```python
from build123d import *

# Parameters (mm, degrees)
F0_W     = 89.995448
F0_H     = 99.06
F1_DEPTH = 38.1
F2_W     = 75.08048
F2_H     = 20.982087
F2_H_2   = 20.982086
F3_DEPTH = 38.1
F4_R     = 5.08
F5_W     = 59.154313
F5_H     = 38.1
F6_DEPTH = 10.16
F7_R     = 5.08
F8_W     = 63.199052
F8_H     = 38.1
F9_DEPTH = 7.62
F10_R    = 5.08


with BuildPart() as f1:
    # F0 (on Top) → F1 (new body)
    with BuildSketch(Plane.XY):
        with Locations((-3.918344, -0.650048)):
            Rectangle(F0_W, F0_H)
    extrude(amount=F1_DEPTH)

    # F2 (on face) → F3 (cut)
    with BuildSketch(Plane.XY.offset(38.1)):
        with Locations((-4.297534, 23.257251)):
            Rectangle(F2_W, F2_H)
        with Locations((-4.297534, -1.516776)):
            Rectangle(F2_W, F2_H_2)
        with Locations((-4.297534, -25.785215)):
            Rectangle(F2_W, F2_H)
    extrude(amount=-F3_DEPTH, mode=Mode.SUBTRACT)

    # F4
    f4_edges = [f1.edges().sort_by_distance(p)[0] for p in [
        (33.242706, 33.748295, 19.05),
        (33.242706, 8.974267, 19.05),
        (33.242706, -15.294172, 19.05),
        (-41.837774, 33.748295, 19.05),
        (-41.837774, 8.974267, 19.05),
        (-41.837774, -15.294172, 19.05),
        (-41.837774, -36.276259, 19.05),
        (-41.837774, -12.007819, 19.05),
        (-41.837774, 12.766208, 19.05),
        (33.242706, -36.276259, 19.05),
        (33.242706, -12.007819, 19.05),
        (33.242706, 12.766208, 19.05),
    ]]
    fillet(f4_edges, radius=F4_R)

    # F5 (on face) → F6 (cut)
    with BuildSketch(Plane(origin=(0, 48.879952, 0), x_dir=(-1, 0, 0), z_dir=(0, 1, 0))):
        with Locations((3.412747, 19.05)):
            Rectangle(F5_W, F5_H)
    extrude(amount=-F6_DEPTH, mode=Mode.SUBTRACT)

    # F7
    f7_edges = [f1.edges().sort_by_distance(p)[0] for p in [
        (-32.989904, 38.719952, 19.05),
        (26.164409, 38.719952, 19.05),
    ]]
    fillet(f7_edges, radius=F7_R)

    # F8 (on face) → F9 (cut)
    with BuildSketch(Plane.XZ.offset(50.180048)):
        with Locations((-2.907156, 19.05)):
            Rectangle(F8_W, F8_H)
    extrude(amount=-F9_DEPTH, mode=Mode.SUBTRACT)

    # F10
    f10_edges = [f1.edges().sort_by_distance(p)[0] for p in [
        (28.69237, -42.560048, 19.05),
        (-34.506682, -42.560048, 19.05),
    ]]
    fillet(f10_edges, radius=F10_R)


solid = f1.part
```
Source: CAD feature listing. Evaluate the final solid. Frame: model axes, mm. A direction names the side the tool comes from. Round coordinates to 2 decimals unless told otherwise and drop trailing zeros. Write each loop counter-clockwise with the first axis right and the second up, starting at its lowest first coordinate (ties: lowest second). Pieces come first, ordered by that corner, then holes. Notation, with made-up numbers: M -2,75.5 L 25,75.5 A25 ccw 25,95.5 Z; hole C 67.5,51 d10. An arc over 180 degrees is marked long. Answer as a JSON object with one key per item and string values. Group by question number.
(1) Section query A-A on x = 5. Output: boundary loops of the cut face in (y, z).
(2) First-contact query: pin 1 (19 mm diameter, centred on x = 2.5, z = 19, fed in from +Y); pin 2 (19 mm diameter, centred on x = -10, z = 11, fed in from -Y). Flat tips, straight axial feed; report the tip coordinate or a pass-through.
(3) Section query B-B on y = -27. Output: boundary loops of the cut face in (x, z), then the cut area to 3 significant figures.
(4) Ray query, line 1 (Y direction, x = -28, z = 36); line 2 (X direction, y = -1.5, z = 3); line 3 (Y direction, x = -30, z = 29). Return the intervals inside material, ascending. Write a range as [from, to].
(5) Section query C-C on z = 4.5. State how many separate pieces and enclosed holes the cut face has, then the cut area to 3 significant figures.
(6) Mould query, pull axis Y, two halves, no side actions, for faces 5 (the flat face through (-4, -15, 0)), 6 (the flat face through (35, -50.18, 19)), 7 (the flat face through (33.243, -2, 19)). Classes: +Y half, -Y half, draft (parallel to the pull), parting line (faces both ways), or undercut.
(7) Section query D-D on y = 7. Output: boundary loops of the cut face in (x, z).
(8) Reachability of faces 1 (the flat face through (-5, -12.008, 19)), 2 (the flat face through (-3, 38.72, 19)), 3 (the flat face through (41.079, -1, 19)), 4 (the flat face through (28.692, -49, 19)) from +Z, -Z, +X, -X, +Y, -Y: full face, straight path, thin tool, end or side. Return the list, or none.
Computed values:
{
 "1": {"outline": "M -42.56,0 L -36.28,0 L -36.28,38.1 L -42.56,38.1 Z; M -15.29,0 L -12.01,0 L -12.01,38.1 L -15.29,38.1 Z; M 8.97,0 L 12.77,0 L 12.77,38.1 L 8.97,38.1 Z; M 33.75,0 L 38.72,0 L 38.72,38.1 L 33.75,38.1 Z"},
 "2": {"pin 1": "y = 38.72", "pin 2": "y = -42.56"},
 "3": {"outline": "M -48.92,0 L -41.84,0 L -41.84,38.1 L -48.92,38.1 Z; M 33.24,0 L 41.08,0 L 41.08,38.1 L 33.24,38.1 Z", "area": "568 mm^2"},
 "4": {"line 1": "[-42.56, -36.28], [-15.29, -12.01], [8.97, 12.77], [33.75, 38.72]", "line 2": "[-48.92, -41.84], [33.24, 41.08]", "line 3": "[-42.59, -36.28], [-15.29, -12.01], [8.97, 12.77], [33.75, 39.17]"},
 "5": {"separate pieces": "1", "enclosed holes": "3", "area": "3,190 mm^2"},
 "6": {"face 5": "draft", "face 6": "-Y half", "face 7": "undercut"},
 "7": {"outline": "M -48.92,0 L -40.78,0 L -40.78,38.1 L -48.92,38.1 Z; M 32.18,0 L 41.08,0 L 41.08,38.1 L 32.18,38.1 Z"},
 "8": {"face 1": "+Z, -Z", "face 2": "+Z, -Z, +Y", "face 3": "+Z, -Z, +X, +Y, -Y", "face 4": "+Z, -Z, -Y"}
}
